from build123d import *

# Parameters (mm, degrees)
F1_DEPTH = 600
F3_DEPTH = 600.001
F4_R     = 80
F5_DEPTH = 1600.001
F7_DEPTH = 200.001


with BuildPart() as f1:
    # F0 (on Front) → F1 (new body)
    with BuildSketch(Plane.XZ):
        Polygon((-800, 0), (0, 0), (800, 0), (800, 200), (364.102565, 200), (364.102565, 615.384671), (-435.897435, 615.384671), (-435.897435, 200), (-800, 200), align=None)
    extrude(amount=F1_DEPTH)

    # F2 (on face) → F3 (cut, through all)
    with BuildSketch(Plane.XZ.offset(600)):
        with BuildLine():
            Line((264.102565, 615.384671), (-335.897435, 615.384671))
            ThreePointArc((-335.897435, 615.384671), (-35.897435, 315.384671), (264.102565, 615.384671))
        make_face()
    extrude(amount=-F3_DEPTH, mode=Mode.SUBTRACT)

    # F4 (on face) → F5 (cut, through all)
    with BuildSketch(Plane.YZ.offset(800)):
        with Locations((-300, 450)):
            Circle(F4_R)
    extrude(amount=-F5_DEPTH, mode=Mode.SUBTRACT)

    # F6 (on face) → F7 (cut, through all)
    with BuildSketch(Plane.XY.offset(200)):
        with BuildLine():
            Line((-710, -150), (-710, -450))
            ThreePointArc((-710, -450), (-650, -510), (-590, -450))
            Line((-590, -450), (-590, -150))
            ThreePointArc((-590, -150), (-650, -90), (-710, -150))
        make_face()
        with BuildLine():
            Line((590, -150), (590, -450))
            ThreePointArc((590, -450), (650, -510), (710, -450))
            Line((710, -450), (710, -150))
            ThreePointArc((710, -150), (650, -90), (590, -150))
        make_face()
    extrude(amount=-F7_DEPTH, mode=Mode.SUBTRACT)


solid = f1.part
The listing builds one solid part. Answer for the finished solid, in the listing's coordinates (mm). A direction names the side the tool comes from. Round coordinates to 2 decimals unless told otherwise and drop trailing zeros. Write each loop counter-clockwise with the first axis right and the second up, starting at its lowest first coordinate (ties: lowest second). Pieces come first, ordered by that corner, then holes. Notation, with made-up numbers: (89, 6.25) - (118, 6.25) arc R11 ccw to (118, 19.25) - close; hole circle Ø6 at (-2.5, -31.75). An arc over 180 degrees is marked (long way). Use a Markdown table: item, result. Add a question column.
1. A flat-ended cylindrical pin translates along its axis: P1, Ø8, axis at y = -149, z = 447, coming from the +X side. Find the tip coordinate at first contact, or state that the pin passes through.
2. The part is cut by section B-B (y = -173). Write down the section's boundary in (x, z).
3. The part is cut by section A-A (x = -650). Write down the section's boundary in (y, z).
4. For a pull along Z with two mould halves and no side action, classify faces 4 (the face through (-575, -296, 200)), 5 (the face through (-800, -296, 101)), 6 (the face through (277.26, -317.34, 371.9)) as +Z half, -Z half, draft (parallel to the pull), parting line (faces both ways), or undercut.
5. Consider line 1 (X direction, y = -153, z = 165.5); line 2 (Z direction, x = 307, y = -300); line 3 (Y direction, x = 230, z = 450). Determine where each line is inside the solid, lowest interval first.
6. The part is cut by section C-C (z = 450). Write down the section's boundary in (x, y), and give its area (3 significant figures).
7. The part is cut by section D-D (z = 140). Write down the section's boundary in (x, y).
8. A tool of negligible diameter and unlimited length cuts with its end or side. For faces 1 (the face through (585, -296, 200)), 2 (the face through (-435.897, -296, 364)), 3 (the face through (-651.319, -509.985, 101.4)), from which of +Z, -Z, +X, -X, +Y, -Y can it reach the whole face along a straight path? Write none if from no direction.
Reported:
| question | item | result |
|---|---|---|
| 1 | P1 | x = 364.1 |
| 2 | outline | (-800, 0) - (-710, 0) - (-710, 200) - (-800, 200) - close; (-590, 0) - (590, 0) - (590, 200) - (364.1, 200) - (364.1, 615.38) - (264.1, 615.38) arc R300 cw to (-335.9, 615.38) - (-435.9, 615.38) - (-435.9, 200) - (-590, 200) - close; (710, 0) - (800, 0) - (800, 200) - (710, 200) - close |
| 3 | outline | (-600, 0) - (-510, 0) - (-510, 200) - (-600, 200) - close; (-90, 0) - (0, 0) - (0, 200) - (-90, 200) - close |
| 4 | face 4 | +Z half |
| 4 | face 5 | draft |
| 4 | face 6 | undercut |
| 5 | line 1 | -800 to -710, -590 to 590, 710 to 800 |
| 5 | line 2 | 0 to 370, 530 to 615.38 |
| 5 | line 3 | -600 to -380, -220 to 0 |
| 6 | outline | (-435.9, -600) - (-286.19, -600) - (-286.19, -380) - (-435.9, -380) - close; (-435.9, -220) - (-286.19, -220) - (-286.19, 0) - (-435.9, 0) - close; (214.4, -600) - (364.1, -600) - (364.1, -380) - (214.4, -380) - close; (214.4, -220) - (364.1, -220) - (364.1, 0) - (214.4, 0) - close |
| 6 | area | 132,000 mm^2 |
| 7 | outline | (-800, -600) - (800, -600) - (800, 0) - (-800, 0) - close; hole (-710, -450) arc R60 ccw to (-590, -450) - (-590, -150) arc R60 ccw to (-710, -150) - close; hole (590, -450) arc R60 ccw to (710, -450) - (710, -150) arc R60 ccw to (590, -150) - close |
| 8 | face 1 | +Z, +X, +Y, -Y |
| 8 | face 2 | +Z, -X, +Y, -Y |
| 8 | face 3 | +Z, -Z |
